Design review of the part built by this model. Coordinates are the model's own, in mm. A direction names the side the tool comes from. Give positions to 0.01 mm unless a question says otherwise; leave off trailing zeros. Write each loop counter-clockwise with the first axis right and the second up, starting at its lowest first coordinate (ties: lowest second). Pieces come first, ordered by that corner, then holes. Notation, with made-up numbers: (21.5, 74.25) - (54.5, 74.25) arc R14 ccw to (54.5, 90.25) - close; hole circle Ø5 at (50, -28.75). An arc over 180 degrees is marked (long way). Use a Markdown table: item, result. Add a question column.
```python
from build123d import *

# Parameters (mm, degrees)
F0_R     = 4
F1_DEPTH = 15
F2_DEPTH = 12
F3_SIZE  = 2


with BuildPart() as f1:
    # F0 (on Top) → F1 (new body)
    with BuildSketch(Plane.XY):
        with BuildLine():
            Line((0, 15), (0, 20.764023))
            Line((0, 20.764023), (-23.369339, 20.764023))
            ThreePointArc((-23.369339, 20.764023), (-26.904873, 19.299557), (-28.369339, 15.764023))
            Line((-28.369339, 15.764023), (-28.369339, -6.304249))
            Line((-28.369339, -6.304249), (0, -6.304249))
            Line((0, -6.304249), (0, 0))
            Line((0, 0), (-10, 0))
            ThreePointArc((-10, 0), (-13.535534, 1.464466), (-15, 5))
            Line((-15, 5), (-15, 10))
            ThreePointArc((-15, 10), (-13.535534, 13.535534), (-10, 15))
            Line((-10, 15), (0, 15))
        make_face()
        with Locations((-22, 0)):
            Circle(F0_R, mode=Mode.SUBTRACT)
        with Locations((-22, 15)):
            Circle(F0_R, mode=Mode.SUBTRACT)
        with BuildLine():
            Line((23.369339, 20.764023), (0, 20.764023))
            Line((0, 20.764023), (0, 15))
            Line((0, 15), (10, 15))
            ThreePointArc((10, 15), (13.535534, 13.535534), (15, 10))
            Line((15, 10), (15, 5))
            ThreePointArc((15, 5), (13.535534, 1.464466), (10, 0))
            Line((10, 0), (0, 0))
            Line((0, 0), (0, -6.304249))
            Line((0, -6.304249), (28.369339, -6.304249))
            Line((28.369339, -6.304249), (28.369339, 15.764023))
            ThreePointArc((28.369339, 15.764023), (26.904873, 19.299557), (23.369339, 20.764023))
        make_face()
        with Locations((22, 0)):
            Circle(F0_R, mode=Mode.SUBTRACT)
        with Locations((22, 15)):
            Circle(F0_R, mode=Mode.SUBTRACT)
        with Locations((-22, 15)):
            Circle(F0_R)
        with Locations((-22, 0)):
            Circle(F0_R)
        with Locations((22, 15)):
            Circle(F0_R)
        with Locations((22, 0)):
            Circle(F0_R)
    extrude(amount=F1_DEPTH)

    # F0 (on Top) → F2 (cut)
    with BuildSketch(Plane.XY):
        with Locations((22, 15)):
            Circle(F0_R)
        with Locations((22, 0)):
            Circle(F0_R)
        with Locations((-22, 15)):
            Circle(F0_R)
        with Locations((-22, 0)):
            Circle(F0_R)
    extrude(amount=F2_DEPTH, mode=Mode.SUBTRACT)

    # F3
    f3_edges = [f1.edges().sort_by_distance(p)[0] for p in [
        (0, 15, 0),
    ]]
    chamfer(f3_edges, length=F3_SIZE)


solid = f1.part
```
(1) Add section A-A (z = 14). State the section outline as (x, y) points.
(2) Tool access review of faces 5 (the face through (0, -2, 15)), 6 (the face through (-16, 7, 1)), 7 (the face through (14, 2, 8)): name each direction out of +Z, -Z, +X, -X, +Y, -Y from which nothing blocks a thin tool from reaching the whole face with its end or side.
(3) Add section D-D (y = -3). State the section outline as (x, z) points, and give its area (3 significant figures).
(4) Mouldability with a two-part tool opening along X and no side actions: class faces 1 (the face through (19.05, 17.7, 5.92)), 2 (the face through (-28.369, 5, 7)), 3 (the face through (-22, 0, 12)), 4 (the face through (28.369, 5, 7)) as +X half, -X half, draft (parallel to the pull), parting line (faces both ways), or undercut.
(5) Add section C-C (x = 22). State the section outline as (y, z) points, and give its area (3 significant figures).
(6) For line 1 along Y through (x, z) = (22, 4.5); line 2 along Y through (x, z) = (1, 14); line 3 along Y through (x, z) = (-18.5, 10.25), list the stretches that pass through material, from the lowest coordinate up.
(7) Insertion check: pin 1 (12 mm diameter, centred on x = 9.5, y = 6, fed in from -Z); pin 2 (2.5 mm diameter, centred on x = 21.5, y = 0.5, fed in from -Z); pin 3 (6 mm diameter, centred on x = 2, y = 1.5, fed in from -Z). Each pin has a flat end and moves straight along its axis. Give the tip position at first contact, or say it passes through.
(8) Add section B-B (y = 6). State the section outline as (x, z) points, and give its area (3 significant figures).
Answers follow:
| question | item | result |
|---|---|---|
| 1 | outline | (-28.37, -6.3) - (28.37, -6.3) - (28.37, 15.76) arc R5 ccw to (23.37, 20.76) - (-23.37, 20.76) arc R5 ccw to (-28.37, 15.76) - close; hole (-15, 5) arc R5 ccw to (-10, 0) - (10, 0) arc R5 ccw to (15, 5) - (15, 10) arc R5 ccw to (10, 15) - (-10, 15) arc R5 ccw to (-15, 10) - close |
| 2 | face 5 | +Z, +X, -X, +Y, -Y |
| 2 | face 6 | -Z |
| 2 | face 7 | +Z, -Z |
| 3 | outline | (-28.37, 0) - (-24.65, 0) - (-24.65, 12) - (-19.35, 12) - (-19.35, 0) - (19.35, 0) - (19.35, 12) - (24.65, 12) - (24.65, 0) - (28.37, 0) - (28.37, 15) - (-28.37, 15) - close |
| 3 | area | 724 mm^2 |
| 4 | face 1 | undercut |
| 4 | face 2 | -X half |
| 4 | face 3 | undercut |
| 4 | face 4 | +X half |
| 5 | outline | (-6.3, 0) - (-4, 0) - (-4, 12) - (4, 12) - (4, 0) - (11, 0) - (11, 12) - (19, 12) - (19, 0) - (20.76, 0) - (20.76, 15) - (-6.3, 15) - close |
| 5 | area | 214 mm^2 |
| 6 | line 1 | -6.3 to -4, 4 to 11, 19 to 20.76 |
| 6 | line 2 | -6.3 to 0, 15 to 20.76 |
| 6 | line 3 | -6.3 to -1.94, 1.94 to 13.06, 16.94 to 20.76 |
| 7 | pin 1 | z = 1.5 |
| 7 | pin 2 | z = 12 |
| 7 | pin 3 | z = 0.5 |
| 8 | outline | (-28.37, 0) - (-17, 0) - (-15, 2) - (-15, 15) - (-28.37, 15) - close; (15, 2) - (17, 0) - (28.37, 0) - (28.37, 15) - (15, 15) - close |
| 8 | area | 397 mm^2 |
